Geometry: final body of the model. Coordinates: model frame, mm. Face numbers are marked on the shaded views. A direction names the side the tool comes from. Give positions to 0.01 mm unless a question says otherwise; leave off trailing zeros. Loops run counter-clockwise (first coordinate to the right, second up) from the corner with the lowest first, then second, coordinate; pieces in that order, holes last. Notation, with made-up numbers: (65.25, 11.25) - (88.25, 11.25) arc R14 ccw to (88.25, 36.25) - close; hole circle Ø10 at (66, 11.25). An arc over 180 degrees is marked (long way). Answer in a Markdown table with one row per item.
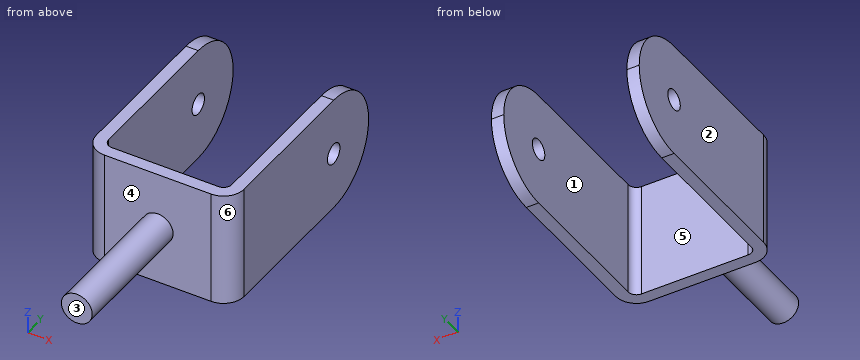
from build123d import *

# Parameters (mm, degrees)
BOSS_EXTRUDE1_DEPTH = 140
FILLET1_R           = 140
SKETCH2_R           = 25
CUT_EXTRUDE1_DEPTH  = 648.765389628
SKETCH3_R           = 37.5
BOSS_EXTRUDE2_DEPTH = 325
FILLET2_R           = 20
FILLET3_R           = 50


with BuildPart() as part:
    # Sketch1 → Boss-Extrude1 (new, symmetric)
    with BuildSketch(Plane.XY):
        Polygon((-150, 0), (150, 0), (150, 520), (180, 520), (180, -30), (-180, -30), (-180, 520), (-150, 520), align=None)
    extrude(amount=BOSS_EXTRUDE1_DEPTH, both=True)

    # Fillet1
    fillet1_edges = [part.edges().sort_by_distance(p)[0] for p in [
        (165, 520, 140),
        (165, 520, -140),
        (-165, 520, -140),
        (-165, 520, 140),
    ]]
    fillet(fillet1_edges, radius=FILLET1_R - 0.0001)  # a hair under: the kernel refuses the full size

    # Sketch2 → Cut-Extrude1 (cut, through all)
    with BuildSketch(Plane(origin=(180, 0, 0), x_dir=(0, 0, -1), z_dir=(1, 0, 0))):
        with Locations((0, 380)):
            Circle(SKETCH2_R)
    extrude(amount=-CUT_EXTRUDE1_DEPTH, mode=Mode.SUBTRACT)

    # Sketch3 → Boss-Extrude2 (add)
    with BuildSketch(Plane.XZ.offset(30)):
        with Locations(Location((0, 0, 0), (0, 0, 270))):
            Circle(SKETCH3_R)
    extrude(amount=BOSS_EXTRUDE2_DEPTH)

    # Fillet2
    fillet2_edges = [part.edges().sort_by_distance(p)[0] for p in [
        (-150, 0, 0),
        (150, 0, 0),
    ]]
    fillet(fillet2_edges, radius=FILLET2_R)

    # Fillet3
    fillet3_edges = [part.edges().sort_by_distance(p)[0] for p in [
        (180, -30, 0),
        (-180, -30, 0),
    ]]
    fillet(fillet3_edges, radius=FILLET3_R)


solid = part.part
Q1. Cut plane D-D (y = 431). Output: boundary loops of the cut face in (x, z), and give its area (3 significant figures).
Check values:
| item | result |
|---|---|
| outline | (-180, -130.38) - (-150, -130.38) - (-150, 130.38) - (-180, 130.38) - close; (150, -130.38) - (180, -130.38) - (180, 130.38) - (150, 130.38) - close |
| area | 15,600 mm² |
Q2. Cut plane A-A (y = 327). Output: boundary loops of the cut face in (x, z), and give its area (3 significant figures).
Check values:
| item | result |
|---|---|
| outline | (-180, -140) - (-150, -140) - (-150, 140) - (-180, 140) - close; (150, -140) - (180, -140) - (180, 140) - (150, 140) - close |
| area | 16,800 mm² |
Q3. Cut plane B-B (x = 0). Output: boundary loops of the cut face in (y, z).
Check values:
| item | result |
|---|---|
| outline | (-355, -37.5) - (-30, -37.5) - (-30, -140) - (0, -140) - (0, 140) - (-30, 140) - (-30, 37.5) - (-355, 37.5) - close |
Q4. Material intervals for line 1 along X through (y, z) = (222.5, 44.5); line 2 along Y through (x, z) = (-121, -70); line 3 along Y through (x, z) = (-160.5, -5.5), sorted ascending.
Check values:
| item | result |
|---|---|
| line 1 | -180 to -150, 150 to 180 |
| line 2 | -30 to 0 |
| line 3 | -19.62 to 355.61, 404.39 to 519.89 |
Q5. First-contact query: pin 1 (6 mm diameter, centred on x = 17.5, z = 30.5, fed in from +Y). Flat tip, straight axial feed; report the tip coordinate or a pass-through.
Check values:
| item | result |
|---|---|
| pin 1 | y = 0 |
Q6. Cut plane C-C (z = 88). Output: boundary loops of the cut face in (x, y).
Check values:
| item | result |
|---|---|
| outline | (-180, 20) arc R50 ccw to (-130, -30) - (130, -30) arc R50 ccw to (180, 20) - (180, 488.89) - (150, 488.89) - (150, 20) arc R20 cw to (130, 0) - (-130, 0) arc R20 cw to (-150, 20) - (-150, 488.89) - (-180, 488.89) - close |
Q7. Reachability of the marked faces 4, 5 and 6 from +Z, -Z, +X, -X, +Y, -Y: full face, straight path, thin tool, end or side. Return the list, or none.
Check values:
| item | result |
|---|---|
| face 4 | -Y |
| face 5 | +Z, -Z, +Y |
| face 6 | +Z, -Z, +X, -Y |
Q8. Draft query along X for the marked faces 1, 2 and 3. Return one class per face: pulls with the +X half, pulls with the -X half, needs draft (parallel to the pull), parting line crosses it, or undercut.
Check values:
| item | result |
|---|---|
| face 1 | undercut |
| face 2 | pulls with the -X half |
| face 3 | needs draft |
